from build123d import *

# Parameters (mm, degrees)
ENL_V_MAT_EXTRU_1_REACH = 10.67
ESQUISSE3_W             = 0.7
ESQUISSE3_H             = 0.7
BOSS_EXTRU_1_DEPTH      = 24.5
ENL_V_START             = -3.3
ENL_V_MAT_EXTRU_2_DEPTH = 5.9
SKETCH1_W               = 4.51
SKETCH1_H               = 19.5
CUT_EXTRUDE1_DEPTH      = 34.394647775


with BuildPart() as part:
    # Esquisse1 → Révolution1 (revolve)
    with BuildSketch(Plane.XY):
        with BuildLine():
            Line((2.5, 7.6), (2.5, 2.5))
            ThreePointArc((2.5, 2.5), (1.767766953, 0.732233047), (0, 0))
            Line((0, 0), (0, 8.6))
            Line((0, 8.6), (2.95, 8.6))
            Line((2.95, 8.6), (2.95, 7.6))
            Line((2.95, 7.6), (2.5, 7.6))
        make_face()
    revolve(axis=Axis((0, 0, 0), (0, 1, 0)))

    # Esquisse2 → Enlèv. mat.-Extru.1 (cut, up to next)
    with BuildSketch(Plane(origin=(0, 7.6, 0), x_dir=(-1, 0, 0), z_dir=(0, -1, 0)), mode=Mode.PRIVATE) as enl_v_mat_extru_1_sk1:
        Polygon((2.031643218, 2.5), (-2.119175806, 2.5), (-0.304277426, 5.41579693), align=None)
    enl_v_mat_extru_1_tool1 = extrude(enl_v_mat_extru_1_sk1.sketch, amount=-ENL_V_MAT_EXTRU_1_REACH, mode=Mode.PRIVATE) & part.part
    add(enl_v_mat_extru_1_tool1.solids().sort_by_distance((0.130603, 7.6, -3.471932))[0], mode=Mode.SUBTRACT)

    # Esquisse3 → Boss.-Extru.1 (add)
    with BuildSketch(Plane(origin=(0, 8.6, 0), x_dir=(1, 0, 0), z_dir=(0, 1, 0))):
        with Locations((0, 1.905)):
            Rectangle(ESQUISSE3_W, ESQUISSE3_H)
        with Locations((0, -0.635)):
            Rectangle(ESQUISSE3_W, ESQUISSE3_H)
        with Locations((0, -1.905)):
            Rectangle(ESQUISSE3_W, ESQUISSE3_H)
        with Locations((0, 0.635)):
            Rectangle(ESQUISSE3_W, ESQUISSE3_H)
    extrude(amount=BOSS_EXTRU_1_DEPTH)

    # Esquisse4 → Enlèv. mat.-Extru.2 (cut)
    with BuildSketch(Plane.ZY.offset(0.35).offset(ENL_V_START)):
        Polygon((-2.885095567, 30.6), (-1.265657514, 30.6), (-1.265657514, 33.921907916), (0, 33.921907916), (0, 31.83), (1.344412991, 31.83), (1.344412991, 30.6), (2.897512796, 30.6), (2.897512796, 34.676886987), (-2.885095567, 34.676886987), align=None)
    extrude(amount=ENL_V_MAT_EXTRU_2_DEPTH, mode=Mode.SUBTRACT)

    # Sketch1 → Cut-Extrude1 (cut, through all)
    with BuildSketch(Plane.ZY.offset(0.35)):
        with Locations((0, 23.35)):
            Rectangle(SKETCH1_W, SKETCH1_H)
    extrude(amount=-CUT_EXTRUDE1_DEPTH, mode=Mode.SUBTRACT)


solid = part.part
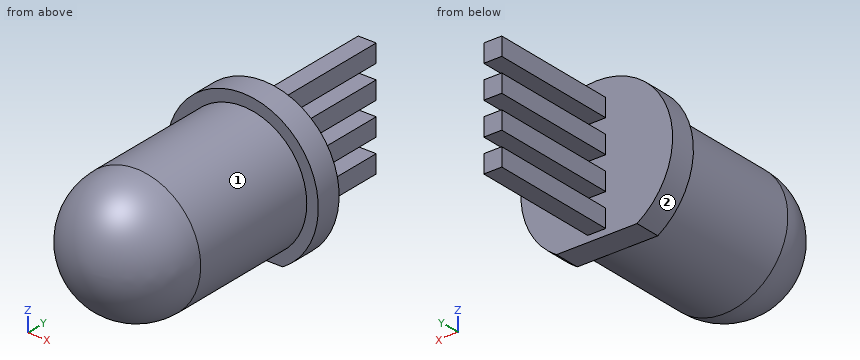
The listing builds one solid part. Answer for the finished solid, in the listing's coordinates (mm). Face numbers are marked on the shaded views. A direction names the side the tool comes from. Round coordinates to 2 decimals unless told otherwise and drop trailing zeros. Order: outer loops, then holes, each group sorted by start corner. A loop starts at its lowest first (then second) coordinate and runs counter-clockwise, first axis right, second up. Notation, with made-up numbers: (54, -3) -> (108, -3) arc R15 ccw to (108, 17) -> close; hole circle Ø6 at (-36.5, 82.25). An arc over 180 degrees is marked (long way). Write each question's results on one line, items separated by ' | '. Start each with the question number.
Q1. Which of the six approach directions +Z, -Z, +X, -X, +Y, -Y give full straight-line access (tool end or side, diameter ignored) to the marked faces 1 and 2?
Q2. Find section B-B (x = -1.95). Determine the outline of the cut face in (y, z).
Q3. Find section D-D (z = -1.85). Determine the outline of the cut face in (x, y), then the cut area to 3 significant figures.
Q4. Each of these flat-tipped pins is pushed along its axis until it touches: pin 1 (0.8 mm diameter, centred on y = 11, z = 1, fed in from -X); pin 2 (0.8 mm diameter, centred on x = 0, y = 10, fed in from -Z) (3 decimals); pin 3 (2 mm diameter, centred on x = -2.5, y = 2, fed in from -Z). Where does it stop, or does it pass through?
Q5. Straight lines are drawn through the part: probe 1 along X at (y, z) = (9.5, 2.15); probe 2 along Y at (x, z) = (2.7, -0.15); probe 3 along X at (y, z) = (2.5, 0.2). For each, find the intervals that lie inside material, in ascending order. Write a range as from..to.
Q6. Find section A-A (z = 0). Determine the outline of the cut face in (x, y).
Q7. Find section C-C (y = 8). Determine the outline of the cut face in (x, z).
Worked answers:
1) face 1: -Y | face 2: +Y, -Y
2) outline: (2.5, -1.56) -> (7.6, -1.56) -> (7.6, -2.21) -> (8.6, -2.21) -> (8.6, 2.21) -> (7.6, 2.21) -> (7.6, 1.56) -> (2.5, 1.56) arc R1.56 ccw to start
3) outline: (-2.3, 7.6) -> (-1.68, 7.6) -> (-1.68, 2.5) arc R1.68 ccw to (1.68, 2.5) -> (1.68, 7.6) -> (2.3, 7.6) -> (2.3, 8.6) -> (0.35, 8.6) -> (0.35, 13.6) -> (-0.35, 13.6) -> (-0.35, 8.6) -> (-2.3, 8.6) -> close | area: 29.7 mm2
4) pin 1: stops at x = -0.35 | pin 2: stops at z = -2.255 | pin 3: stops at z = -1.96
5) probe 1: x = -0.35..0.35 | probe 2: y = 7.6..8.6 | probe 3: x = -2.49..2.49
6) outline: (-2.95, 7.6) -> (-2.5, 7.6) -> (-2.5, 2.5) arc R2.5 ccw to (2.5, 2.5) -> (2.5, 7.6) -> (2.95, 7.6) -> (2.95, 8.6) -> (-2.95, 8.6) -> close
7) outline: (-1.57, -2.5) -> (1.57, -2.5) arc R2.95 ccw (long way) to start
